CAD build for the part. Positions are in the model's coordinates, mm. Coordinates: 2 decimals unless noted, no trailing zeros. Answer in a Markdown table with one row per item. Add a question column.
Q1. Pin check, flat tips, straight feed: pin 1 (0.6 mm diameter, centred on x = -2.5, z = 1.5, fed in from -Y); pin 2 (1.6 mm diameter, centred on y = 84.5, z = 2, fed in from -X); pin 3 (1 mm diameter, centred on x = -4, z = 2, fed in from +Y). Stop position of each tip, or through.
Q2. Drill centre lines: line 1 along X through (y, z) = (66, 1.15); line 2 along Y through (x, z) = (0, 2); line 3 along X through (y, z) = (30.5, 2.3). Where is each one in solid material? Low to high. Write a range as from..to.
Q3. Band-saw the part on A-A (z = 1.25). State how many separate pieces and enclosed holes the cut face has, and give its area (3 significant figures).
```python
from build123d import *

# Parameters (mm, degrees)
SKETCH3_W           = 180
SKETCH3_H           = 180
SKETCH3_R           = 1
SKETCH3_R_2         = 1.59
BOSS_EXTRUDE1_DEPTH = 3.18
CUT_EXTRUDE1_DEPTH  = 128.318939675
SKETCH5_R           = 1.436023081
SKETCH5_W           = 3.18
SKETCH5_H           = 80.125
CUT_EXTRUDE2_DEPTH  = 128.318939675


with BuildPart() as part:
    # Sketch3 → Boss-Extrude1 (new body)
    with BuildSketch(Plane.XY):
        Rectangle(SKETCH3_W, SKETCH3_H)
        with Locations(Location((-11.39889268, -5.07556396, 0), (0, 0, 180))):
            Circle(SKETCH3_R, mode=Mode.SUBTRACT)
        with Locations(Location((30.80110732, -22.57556396, 0), (0, 0, 180))):
            Circle(SKETCH3_R, mode=Mode.SUBTRACT)
        with Locations(Location((73.5, 33.341660125, 0), (0, 0, 180))):
            Circle(SKETCH3_R_2, mode=Mode.SUBTRACT)
        with Locations(Location((21.1, 38.441660125, 0), (0, 0, 180))):
            Circle(SKETCH3_R_2, mode=Mode.SUBTRACT)
        with Locations(Location((21.1, 66.341660125, 0), (0, 0, 180))):
            Circle(SKETCH3_R_2, mode=Mode.SUBTRACT)
        with Locations(Location((71.9, 81.641660125, 0), (0, 0, 180))):
            Circle(SKETCH3_R_2, mode=Mode.SUBTRACT)
    extrude(amount=BOSS_EXTRUDE1_DEPTH)

    # Sketch4 → Cut-Extrude1 (cut, through all)
    with BuildSketch(Plane.XY.offset(3.18)):
        Polygon((1.5, 86.82), (10, 86.82), (10, 90), (-10, 90), (-10, 86.82), (-1.5, 86.82), (-1.5, 82.82), (-3.5, 82.82), (-3.5, 79.82), (-1.5, 79.82), (-1.5, 77), (1.5, 77), (1.5, 79.82), (3.5, 79.82), (3.5, 82.82), (1.5, 82.82), align=None)
        Polygon((1.5, -79.82), (1.5, -77), (-1.5, -77), (-1.5, -79.82), (-3.5, -79.82), (-3.5, -82.82), (-1.5, -82.82), (-1.5, -86.82), (-10, -86.82), (-10, -90), (10, -90), (10, -86.82), (1.5, -86.82), (1.5, -82.82), (3.5, -82.82), (3.5, -79.82), align=None)
    extrude(amount=-CUT_EXTRUDE1_DEPTH, mode=Mode.SUBTRACT)

    # Sketch5 → Cut-Extrude2 (cut, through all)
    with BuildSketch(Plane.XY.offset(3.18)):
        with Locations((-88, 0)):
            Circle(SKETCH5_R)
        with Locations((88, 0)):
            Circle(SKETCH5_R)
        with Locations((-88.41, 49.9375)):
            Rectangle(SKETCH5_W, SKETCH5_H)
        with Locations((-88.41, -49.9375)):
            Rectangle(SKETCH5_W, SKETCH5_H)
        with Locations((88.41, -49.9375)):
            Rectangle(SKETCH5_W, SKETCH5_H)
        with Locations((88.41, 49.9375)):
            Rectangle(SKETCH5_W, SKETCH5_H)
    extrude(amount=-CUT_EXTRUDE2_DEPTH, mode=Mode.SUBTRACT)


solid = part.part
```
Checked values:
| question | item | result |
|---|---|---|
| 1 | pin 1 | stops at y = -86.82 |
| 1 | pin 2 | stops at x = -86.82 |
| 1 | pin 3 | stops at y = 86.82 |
| 2 | line 1 | x = -86.82..19.55, 22.65..86.82 |
| 2 | line 2 | y = -77..77 |
| 2 | line 3 | x = -86.82..86.82 |
| 3 | separate pieces | 1 |
| 3 | enclosed holes | 8 |
| 3 | area | 31,100 mm² |
